The model under review builds one solid part; all positions refer to its coordinate system, in mm. Coordinates: 2 decimals unless noted, no trailing zeros. Order: outer loops, then holes, each group sorted by start corner. A loop starts at its lowest first (then second) coordinate and runs counter-clockwise, first axis right, second up. Notation, with made-up numbers: M -14.75,51 L 20.25,51 A26 ccw 20.25,88 Z; hole C 21,76.25 d2. An arc over 180 degrees is marked long. Answer in a Markdown table with one row per item.
from build123d import *

# Parameters (mm, degrees)
SKETCH1_R           = 6.35
BOSS_EXTRUDE1_DEPTH = 6.35


with BuildPart() as part:
    # Sketch1 → Boss-Extrude1 (new body)
    with BuildSketch(Plane(origin=(0, 0, 0), x_dir=(1, 0, 0), z_dir=(0, 1, 0))):
        with BuildLine():
            Line((76.2, -152.4), (25.106996492, 7.99757633))
            ThreePointArc((25.106996492, 7.99757633), (0, 26.35), (-25.106996492, 7.99757633))
            Line((-25.106996492, 7.99757633), (-76.2, -152.4))
            Line((-76.2, -152.4), (-76.2, -203.2))
            Line((-76.2, -203.2), (152.4, -203.2))
            Line((152.4, -203.2), (152.4, -152.4))
            Line((152.4, -152.4), (76.2, -152.4))
        make_face()
        Circle(SKETCH1_R, mode=Mode.SUBTRACT)
    extrude(amount=BOSS_EXTRUDE1_DEPTH)


solid = part.part
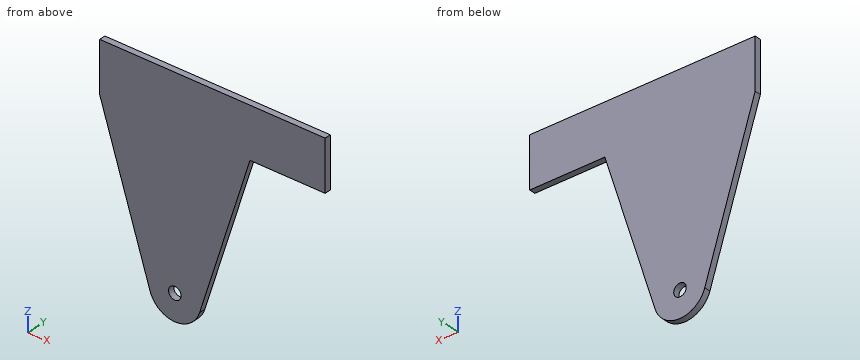
(1) Insertion check: P1, Ø1.9, axis at x = 117.5, y = 2, coming from the -Z side. The pin has a flat end and moves straight along its axis. Give the tip position at first contact, or say it passes through.
Report:
| item | result |
|---|---|
| P1 | z = 152.4 |
(2) Take a section at C-C (y = 3.75). Write out the cut boundary in (x, z), then the cut area to 3 significant figures.
Report:
| item | result |
|---|---|
| outline | M -76.2,152.4 L -25.11,-8 A26.35 ccw 25.11,-8 L 76.2,152.4 L 152.4,152.4 L 152.4,203.2 L -76.2,203.2 Z; hole C 0,0 d12.7 |
| area | 28,400 mm^2 |
(3) To check wall thickness, follow line 1 (Z direction, x = 0, y = 2.5); line 2 (Z direction, x = 89.5, y = 0.75); line 3 (X direction, y = 3.5, z = 0). State the ranges of each line that lie inside material, in increasing order. Write a range as [from, to].
Report:
| item | result |
|---|---|
| line 1 | [-26.35, -6.35], [6.35, 203.2] |
| line 2 | [152.4, 203.2] |
| line 3 | [-27.65, -6.35], [6.35, 27.65] |
(4) Take a section at A-A (x = 0). Write out the cut boundary in (y, z).
Report:
| item | result |
|---|---|
| outline | M 0,-26.35 L 6.35,-26.35 L 6.35,-6.35 L 0,-6.35 Z; M 0,6.35 L 6.35,6.35 L 6.35,203.2 L 0,203.2 Z |
(5) Take a section at D-D (x = 112). Write out the cut boundary in (y, z).
Report:
| item | result |
|---|---|
| outline | M 0,152.4 L 6.35,152.4 L 6.35,203.2 L 0,203.2 Z |
(6) Take a section at B-B (z = 0). Write out the cut boundary in (x, y), then the cut area to 3 significant figures.
Report:
| item | result |
|---|---|
| outline | M -27.65,0 L -6.35,0 L -6.35,6.35 L -27.65,6.35 Z; M 6.35,0 L 27.65,0 L 27.65,6.35 L 6.35,6.35 Z |
| area | 271 mm^2 |
